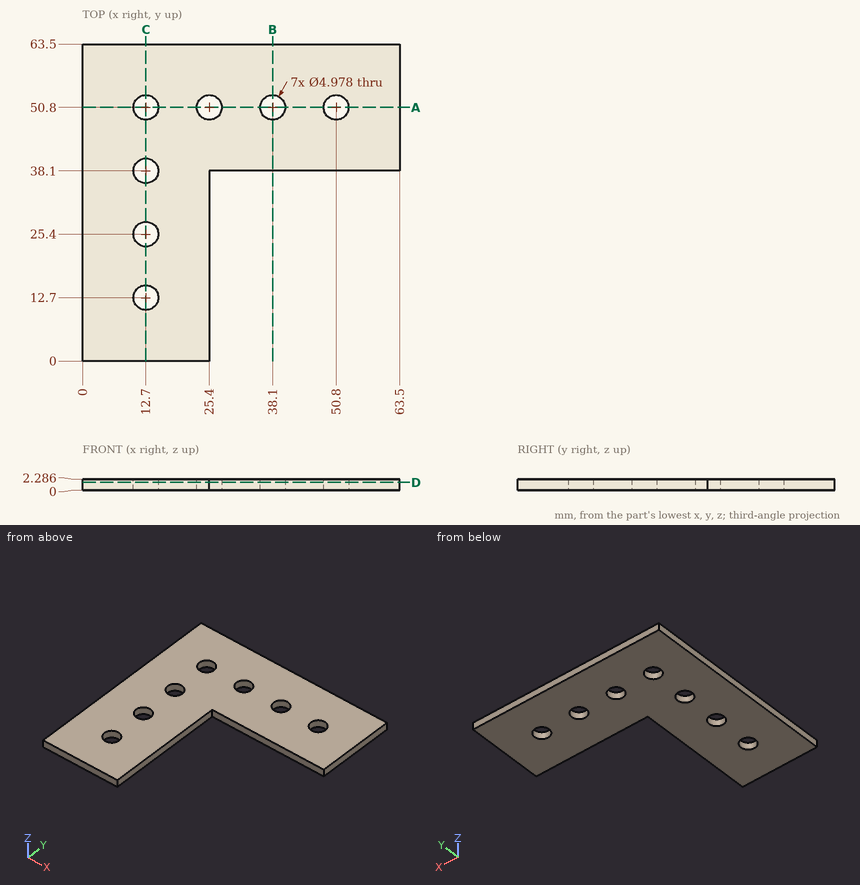
Here's the drawing with two shaded views (mm, measured from the low corner). I have some questions. Give positions to 0.01 mm unless a question says otherwise; leave off trailing zeros. Loops run counter-clockwise (first coordinate to the right, second up) from the corner with the lowest first, then second, coordinate; pieces in that order, holes last. Notation, with made-up numbers: M 43.25,56 L 84.25,56 A31 ccw 84.25,84 Z; hole C -6.75,57 d9. An arc over 180 degrees is marked long. One line per item, written item: value.
1) Please list where these lines run through material, in increasing order: line 1 (X direction, y = 51, z = 0.6); line 2 (Y direction, x = 12.7, z = 1.2); line 3 (X direction, y = 51.5, z = 1.65).
Geometry check:
line 1: x = 0 to 10.22, 15.18 to 22.92, 27.88 to 35.62, 40.58 to 48.32, 53.28 to 63.5
line 2: y = 0 to 10.21, 15.19 to 22.91, 27.89 to 35.61, 40.59 to 48.31, 53.29 to 63.5
line 3: x = 0 to 10.31, 15.09 to 23.01, 27.79 to 35.71, 40.49 to 48.41, 53.19 to 63.5
2) Imagine slicing it at D-D on z = 1.6. Write out the boundary of the cut face in (x, y).
Geometry check:
outline: M 0,0 L 25.4,0 L 25.4,38.1 L 63.5,38.1 L 63.5,63.5 L 0,63.5 Z; hole C 12.7,12.7 d4.98; hole C 12.7,25.4 d4.98; hole C 12.7,38.1 d4.98; hole C 12.7,50.8 d4.98; hole C 25.4,50.8 d4.98; hole C 38.1,50.8 d4.98; hole C 50.8,50.8 d4.98
3) Imagine slicing it at A-A on y = 50.8. Write out the boundary of the cut face in (x, z).
Geometry check:
outline: M 0,0 L 10.21,0 L 10.21,2.29 L 0,2.29 Z; M 15.19,0 L 22.91,0 L 22.91,2.29 L 15.19,2.29 Z; M 27.89,0 L 35.61,0 L 35.61,2.29 L 27.89,2.29 Z; M 40.59,0 L 48.31,0 L 48.31,2.29 L 40.59,2.29 Z; M 53.29,0 L 63.5,0 L 63.5,2.29 L 53.29,2.29 Z
4) Imagine slicing it at B-B on x = 38.1. Write out the boundary of the cut face in (y, z).
Geometry check:
outline: M 38.1,0 L 48.31,0 L 48.31,2.29 L 38.1,2.29 Z; M 53.29,0 L 63.5,0 L 63.5,2.29 L 53.29,2.29 Z
5) I'm going to push a flat-ended pin straight in: pin 1 (1 mm diameter, centred on y = 25.5, z = 0.5, fed in from +X). Where does the tip first touch, or does it pass through?
Geometry check:
pin 1: stops at x = 25.4
